```python
from build123d import *

# Parameters (mm, degrees)
SKETCH1_R           = 1.375
BOSS_EXTRUDE1_DEPTH = 10
CHAMFER1_SIZE       = 5
SKETCH2_W           = 8
SKETCH2_H           = 45
BOSS_EXTRUDE2_DEPTH = 55
SKETCH5_R           = 1.375
CUT_EXTRUDE2_DEPTH  = 186.151289491
SKETCH5_3_R         = 2.6
CUT_EXTRUDE3_DEPTH  = 52
SKETCH1_3_R         = 1.375
CUT_EXTRUDE4_DEPTH  = 10
CHAMFER3_SIZE       = 55.077249093
CHAMFER3_SIZE_2     = 45
SKETCH6_R           = 1.375
CUT_EXTRUDE5_DEPTH  = 10


with BuildPart() as part:
    # Sketch1 → Boss-Extrude1 (new body)
    with BuildSketch(Plane.XY):
        Polygon((-50, 110.5), (-50, -110.5), (50, -110.5), (50, 110.5), (29, 110.5), (29, 43.01), (-29, 43.01), (-29, 110.5), align=None)
        with BuildLine():
            ThreePointArc((-42.5, -64.375), (-43.875, -63), (-42.5, -61.625))
            ThreePointArc((-42.5, -61.625), (-41.125, -63), (-42.5, -64.375))
        make_face(mode=Mode.SUBTRACT)
        with Locations((42.5, -63)):
            Circle(SKETCH1_R, mode=Mode.SUBTRACT)
        with BuildLine():
            ThreePointArc((-42.5, 15.875), (-41.125, 14.5), (-42.5, 13.125))
            ThreePointArc((-42.5, 13.125), (-43.875, 14.5), (-42.5, 15.875))
        make_face(mode=Mode.SUBTRACT)
        with Locations((42.5, 14.5)):
            Circle(SKETCH1_R, mode=Mode.SUBTRACT)
    extrude(amount=BOSS_EXTRUDE1_DEPTH)

    # Chamfer1
    chamfer1_edges = [part.edges().sort_by_distance(p)[0] for p in [
        (29, 43.01, 5),
        (-29, 43.01, 5),
    ]]
    chamfer(chamfer1_edges, length=CHAMFER1_SIZE)

    # Sketch2 → Boss-Extrude2 (add)
    with BuildSketch(Plane.XY.offset(10)):
        with Locations((-42.5, -88)):
            Rectangle(SKETCH2_W, SKETCH2_H)
        with Locations((42.5, -88)):
            Rectangle(SKETCH2_W, SKETCH2_H)
    extrude(amount=BOSS_EXTRUDE2_DEPTH)

    # Sketch5 → Cut-Extrude2 (cut, through all)
    with BuildSketch(Plane(origin=(0, -55.5, 0), x_dir=(1, 0, 0), z_dir=(0, 1, 0))):
        with Locations(Location((-42.5, -17.5, 0), (0, 0, 270))):
            Circle(SKETCH5_R)
        with Locations(Location((-42.5, -57.5, 0), (0, 0, 270))):
            Circle(SKETCH5_R)
        with Locations(Location((42.5, -17.5, 0), (0, 0, 270))):
            Circle(SKETCH5_R)
        with Locations(Location((42.5, -57.5, 0), (0, 0, 270))):
            Circle(SKETCH5_R)
    extrude(amount=-CUT_EXTRUDE2_DEPTH, mode=Mode.SUBTRACT)

    # Sketch5<3> → Cut-Extrude3 (cut)
    with BuildSketch(Plane(origin=(0, -55.5, 0), x_dir=(1, 0, 0), z_dir=(0, 1, 0))):
        with Locations(Location((-42.5, -17.5, 0), (0, 0, 270))):
            Circle(SKETCH5_3_R)
        with Locations(Location((-42.5, -57.5, 0), (0, 0, 270))):
            Circle(SKETCH5_3_R)
        with Locations(Location((42.5, -17.5, 0), (0, 0, 180))):
            Circle(SKETCH5_3_R)
        with Locations(Location((42.5, -57.5, 0), (0, 0, 180))):
            Circle(SKETCH5_3_R)
    extrude(amount=-CUT_EXTRUDE3_DEPTH, mode=Mode.SUBTRACT)

    # Sketch1<3> → Cut-Extrude4 (cut)
    with BuildSketch(Plane.XY):
        with Locations((-42.5, -103)):
            Circle(SKETCH1_3_R)
        with Locations(Location((42.5, -103, 0), (0, 0, 180))):
            Circle(SKETCH1_3_R)
    extrude(amount=CUT_EXTRUDE4_DEPTH, mode=Mode.SUBTRACT)

    # Chamfer3
    # the kernel refuses this chamfer: 55.077249093, 45 mm, written as the material it takes off along each edge
    with BuildSketch(Plane(origin=(188.501029674, -65.5, 65), x_dir=(0, 0.02454043401221108, -0.9996988382000312), z_dir=(-1, 0, 0))) as chamfer3_piece_1_section:
        Polygon((CHAMFER3_SIZE * 0.9996988382, CHAMFER3_SIZE * 0.0245404340122), (-CHAMFER3_SIZE_2 * 0.0245404340122, CHAMFER3_SIZE_2 * 0.9996988382), (0, 0), align=None)
    chamfer3_piece_1 = extrude(amount=292.002059347, mode=Mode.PRIVATE)
    chamfer3_piece_1 = split(chamfer3_piece_1, bisect_by=Plane(origin=(42.5, -80.263234933, 10), z_dir=(0, 0, 1)), keep=Keep.TOP, mode=Mode.PRIVATE)
    add(chamfer3_piece_1, mode=Mode.SUBTRACT)
    with BuildSketch(Plane(origin=(103.501029674, -65.5, 65), x_dir=(0, 0.02454043401221108, -0.9996988382000312), z_dir=(-1, 0, 0))) as chamfer3_piece_2_section:
        Polygon((CHAMFER3_SIZE * 0.9996988382, CHAMFER3_SIZE * 0.0245404340122), (-CHAMFER3_SIZE_2 * 0.0245404340122, CHAMFER3_SIZE_2 * 0.9996988382), (0, 0), align=None)
    chamfer3_piece_2 = extrude(amount=292.002059347, mode=Mode.PRIVATE)
    chamfer3_piece_2 = split(chamfer3_piece_2, bisect_by=Plane(origin=(42.5, -80.263234933, 10), z_dir=(0, 0, 1)), keep=Keep.TOP, mode=Mode.PRIVATE)
    add(chamfer3_piece_2, mode=Mode.SUBTRACT)

    # Sketch6 → Cut-Extrude5 (cut)
    with BuildSketch(Plane.XY.offset(10)):
        with Locations((-35, 95.5)):
            Circle(SKETCH6_R)
        with Locations((35, 95.5)):
            Circle(SKETCH6_R)
        with Locations((35, 40.52)):
            Circle(SKETCH6_R)
        with Locations((-35, 40.52)):
            Circle(SKETCH6_R)
    extrude(amount=-CUT_EXTRUDE5_DEPTH, mode=Mode.SUBTRACT)


solid = part.part
```
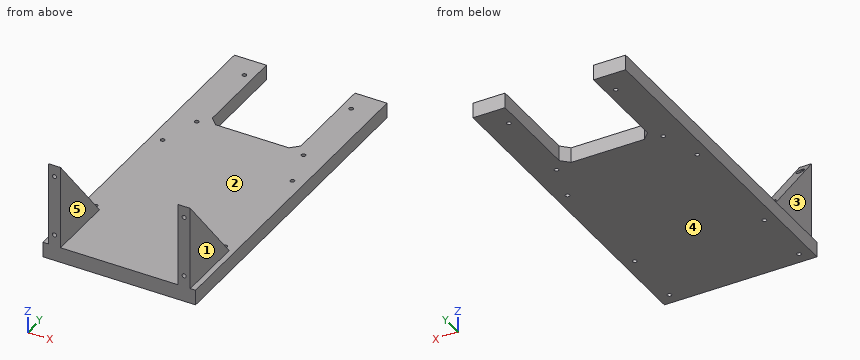
Check sheet for the modelled part. Datum: model origin and axes. Units: mm. Face numbers are marked on the shaded views. A direction names the side the tool comes from. Coordinates: 2 decimals unless noted, no trailing zeros. Loops run counter-clockwise (first coordinate to the right, second up) from the corner with the lowest first, then second, coordinate; pieces in that order, holes last.
1) Access from +Z, -Z, +X, -X, +Y, -Y to the whole of each face (thin tool, end or side, straight path). Record for the marked faces 4 and 5.
2) Sectioned sample at C-C (z = 38). Record the boundary of the cut face in (x, y).
3) Sectioned sample at B-B (y = -83.5). Record the boundary of the cut face in (x, z), and give its area (3 significant figures).
4) Sectioned sample at A-A (z = 6.5). Count the separate pieces of the cut face and the enclosed holes in it, and give its area (3 significant figures).
5) Release check for a two-part mould opening along X. For the marked faces 1, 2 and 3 record: released by +X, released by -X, zero draft, split by the parting line, or undercut.
6) Sectioned sample at D-D (x = -3). Record the boundary of the cut face in (y, z), and give its area (3 significant figures).
7) Gauge pin test, flat ends, axial feed: pin 1 (22.5 mm diameter, centred on y = -89.5, z = 25, fed in from +X); pin 2 (2.5 mm diameter, centred on x = -41, z = 57.5, fed in from +Y); pin 3 (2.5 mm diameter, centred on x = 43, z = 57, fed in from +Y). Record the tip position at first contact, or that the pin passes through.
8) Material ranges on probe 1 along Y at (x, z) = (-35, 7.25) (3 decimals); probe 2 along X at (y, z) = (-109.1, 57.5) (3 decimals); probe 3 along Z at (x, y) = (34.5, -28), recorded low to high.
Check sheet entries:
1. face 4: -Z, +X, -X, +Y, -Y
1. face 5: +Z, +Y, -Y
2. outline: (-46.5, -110.5) - (-38.5, -110.5) - (-38.5, -88.44) - (-46.5, -88.44) - close; (38.5, -110.5) - (46.5, -110.5) - (46.5, -88.44) - (38.5, -88.44) - close
3. outline: (-50, 0) - (50, 0) - (50, 10) - (46.5, 10) - (46.5, 31.95) - (38.5, 31.95) - (38.5, 10) - (-38.5, 10) - (-38.5, 31.95) - (-46.5, 31.95) - (-46.5, 10) - (-50, 10) - close; hole circle Ø5.2 at (-42.5, 17.5); hole circle Ø5.2 at (42.5, 17.5)
3. area: 1,310 mm2
4. separate pieces: 1
4. enclosed holes: 10
4. area: 18,200 mm2
5. face 1: released by +X
5. face 2: undercut
5. face 3: released by -X
6. outline: (-110.5, 0) - (43.01, 0) - (43.01, 10) - (-110.5, 10) - close
6. area: 1,540 mm2
7. pin 1: stops at x = 46.5
7. pin 2: stops at y = -103.74
7. pin 3: stops at y = -107.5
8. probe 1: y = -110.5 to 39.145, 41.895 to 94.125, 96.875 to 110.5
8. probe 2: x = -46.5 to -43.875, -41.125 to -38.5, 38.5 to 41.125, 43.875 to 46.5
8. probe 3: z = 0 to 10
